Could you check a few things on this model? Use its own coordinates, in mm. Coordinates: 2 decimals unless noted, no trailing zeros. Order: outer loops, then holes, each group sorted by start corner. A loop starts at its lowest first (then second) coordinate and runs counter-clockwise, first axis right, second up. Notation, with made-up numbers: (-8.5, 81.25) -> (-0.5, 81.25) arc R8 cw to (-0.5, 90.25) -> close; hole circle Ø11 at (62, -13). An arc over 180 degrees is marked (long way). Use a Markdown table: item, result. Add a question column.
1) If we section it at A-A (z = -8.75): Write out the boundary of the cut face in (x, y).
2) If I drill on L1, parallel to X at y = 0.7, z = -8.75, over which ranges is the centre line in solid material (lowest first)? Write a range as [from, to].
3) If we section it at B-B (y = 0.4): Give the number of separate pieces and of enclosed holes in the cut face, plus the area to 3 significant figures.
4) If we section it at C-C (x = -1.27): Write out the boundary of the cut face in (y, z), plus the area to 3 significant figures.
5) Will this pin go through, and if not, where does the flat tip stop? pin 1 Ø0.9 at (x, z) = (-21, 8.75) entering from +Y.
6) If we section it at D-D (x = 13): Write out the boundary of the cut face in (y, z).
7) Thinking about a two-plate mould opening in X: for faces 1 (the flat face through (0, 0, 0)), 2 (the flat face through (-22.5, 1, 0)), 3 (the cylindrical face through (12.51, 0.76, 5.25)), 4 (the flat face through (22.5, 1, 0)), which applies, +X half, -X half, draft (parallel to the pull), parting line (faces both ways), or undercut?
```python
from build123d import *

# Parameters (mm, degrees)
SKETCH1_W   = 45
SKETCH1_H   = 20
SKETCH1_R   = 0.75
PCB_DEPTH   = 1.5
SKETCH2_R   = 0.5
SKETCH2_R_2 = 0.55
HOLES_DEPTH = 2


with BuildPart() as part:
    # Sketch1 → PCB (new body)
    with BuildSketch(Plane(origin=(0, 0, 0), x_dir=(1, 0, 0), z_dir=(0, 1, 0))):
        Rectangle(SKETCH1_W, SKETCH1_H)
        with Locations(Location((-21, 8.75, 0), (0, 0, 270))):
            Circle(SKETCH1_R, mode=Mode.SUBTRACT)
        with Locations(Location((-21, -8.75, 0), (0, 0, 270))):
            Circle(SKETCH1_R, mode=Mode.SUBTRACT)
        with Locations(Location((21, -8.75, 0), (0, 0, 270))):
            Circle(SKETCH1_R, mode=Mode.SUBTRACT)
        with Locations(Location((21, 8.75, 0), (0, 0, 270))):
            Circle(SKETCH1_R, mode=Mode.SUBTRACT)
    extrude(amount=PCB_DEPTH)

    # Sketch2 → Holes (cut)
    with BuildSketch(Plane(origin=(0, 1.5, 0), x_dir=(1, 0, 0), z_dir=(0, 1, 0))):
        with Locations(Location((-3.81, -8.73, 0), (0, 0, 270))):
            Circle(SKETCH2_R)
        with Locations(Location((-1.27, -8.73, 0), (0, 0, 270))):
            Circle(SKETCH2_R)
        with Locations(Location((1.27, -8.73, 0), (0, 0, 270))):
            Circle(SKETCH2_R)
        with Locations(Location((3.81, -8.73, 0), (0, 0, 270))):
            Circle(SKETCH2_R)
        with Locations(Location((13, 5, 0), (0, 0, 270))):
            Circle(SKETCH2_R_2)
        with Locations(Location((13, -5, 0), (0, 0, 270))):
            Circle(SKETCH2_R_2)
        with Locations(Location((-13, -5, 0), (0, 0, 270))):
            Circle(SKETCH2_R_2)
        with Locations(Location((-13, 5, 0), (0, 0, 270))):
            Circle(SKETCH2_R_2)
    extrude(amount=-HOLES_DEPTH, mode=Mode.SUBTRACT)


solid = part.part
```
Answer sheet:
| question | item | result |
|---|---|---|
| 1 | outline | (-22.5, 0) -> (-21.75, 0) -> (-21.75, 1.5) -> (-22.5, 1.5) -> close; (-20.25, 0) -> (20.25, 0) -> (20.25, 1.5) -> (-20.25, 1.5) -> close; (21.75, 0) -> (22.5, 0) -> (22.5, 1.5) -> (21.75, 1.5) -> close |
| 2 | L1 | [-22.5, -21.75], [-20.25, 20.25], [21.75, 22.5] |
| 3 | separate pieces | 1 |
| 3 | enclosed holes | 12 |
| 3 | area | 886 mm2 |
| 4 | outline | (0, -10) -> (1.5, -10) -> (1.5, 8.23) -> (0, 8.23) -> close; (0, 9.23) -> (1.5, 9.23) -> (1.5, 10) -> (0, 10) -> close |
| 4 | area | 28.5 mm2 |
| 5 | pin 1 | through |
| 6 | outline | (0, -10) -> (1.5, -10) -> (1.5, -5.55) -> (0, -5.55) -> close; (0, -4.45) -> (1.5, -4.45) -> (1.5, 4.45) -> (0, 4.45) -> close; (0, 5.55) -> (1.5, 5.55) -> (1.5, 10) -> (0, 10) -> close |
| 7 | face 1 | draft |
| 7 | face 2 | -X half |
| 7 | face 3 | undercut |
| 7 | face 4 | +X half |
